Check sheet for the modelled part. Datum: model origin and axes. Units: mm. Face numbers are marked on the shaded views. A direction names the side the tool comes from. Round coordinates to 2 decimals unless told otherwise and drop trailing zeros. Write each loop counter-clockwise with the first axis right and the second up, starting at its lowest first coordinate (ties: lowest second). Pieces come first, ordered by that corner, then holes. Notation, with made-up numbers: (12.25, 75) - (31.25, 75) arc R21 ccw to (31.25, 81) - close; hole circle Ø3 at (-36.75, 62). An arc over 180 degrees is marked (long way). Answer as a JSON object with one key per item and string values. Group by question number.
Item 1: Gauge pin test, flat ends, axial feed: P1, Ø1.6, axis at x = -27.5, z = -8, coming from the +Y side; P2, Ø6, axis at x = -60, z = -7.5, coming from the +Y side. Record the tip position at first contact, or that the pin passes through.
Item 2: Release check for a two-part mould opening along X. For the marked faces 1, 2, 3 and 4 record: pulls with the +X half, pulls with the -X half, needs draft (parallel to the pull), parting line crosses it, or undercut.
Item 3: Sectioned sample at C-C on y = 3.75. Count the separate pieces of the cut face and the enclosed holes in it, plus the area to 3 significant figures.
Item 4: Sectioned sample at B-B on x = -7. Record the boundary of the cut face in (y, z), plus the area to 3 significant figures.
Item 5: Thickness scan on line 1 (X direction, y = 5.75, z = -28.5); line 2 (Z direction, x = -66, y = 9.25); line 3 (X direction, y = 7.25, z = -4.5). Record the ranges inside material, lowest first.
Item 6: Sectioned sample at D-D on x = -97. Record the boundary of the cut face in (y, z).
Item 7: Set-up check for the marked faces 5 and 6: record each of +Z, -Z, +X, -X, +Y, -Y from which the full face is reachable in a straight line by a thin tool's end or side.
Item 8: Sectioned sample at A-A on z = -46.4. Record the boundary of the cut face in (x, y).
```python
from build123d import *

# Parameters (mm, degrees)
SKETCH_1_W           = 120
SKETCH_1_H           = 53
EXTRUDE_2_DEPTH      = 16.4
SKETCH_4_W           = 116
SKETCH_4_H           = 49
CUT_EXTRUDE_5_DEPTH  = 15.2
SKETCH_5_W           = 118.4
SKETCH_5_H           = 51.4
CUT_EXTRUDE_6_DEPTH  = 3
SKETCH_6_W           = 57.1
SKETCH_6_H           = 36.3
EXTRUDE_3_DEPTH      = 10.7
SKETCH_7_W           = 55.5
SKETCH_7_H           = 35.5
CUT_EXTRUDE_7_DEPTH  = 10.7
SKETCH_8_W           = 3.401063497
SKETCH_8_H           = 16.4
CUT_EXTRUDE_8_DEPTH  = 10.7
SKETCH_9_R           = 8.9
EXTRUDE_4_DEPTH      = 14
SKETCH_10_R          = 7.7
CUT_EXTRUDE_9_DEPTH  = 14
SKETCH_12_W          = 1.431066628
SKETCH_12_H          = 20
CUT_EXTRUDE_10_DEPTH = 10.7
SKETCH_11_R          = 8
EXTRUDE_8_DEPTH      = 14
SKETCH_13_R          = 6.8
CUT_EXTRUDE_11_DEPTH = 14
SKETCH_14_W          = 22.6
SKETCH_14_H          = 8.7
EXTRUDE_9_DEPTH      = 12.2
SKETCH_15_W          = 21
SKETCH_15_H          = 9.750364289
CUT_EXTRUDE_12_DEPTH = 5.2
SKETCH_16_W          = 16
SKETCH_16_H          = 2
CUT_EXTRUDE_13_DEPTH = 7
SKETCH_18_W          = 21
SKETCH_18_H          = 2
CUT_EXTRUDE_14_DEPTH = 7
SKETCH_19_W          = 20.6
SKETCH_19_H          = 8.7
EXTRUDE_10_DEPTH     = 12.2
SKETCH_21_W          = 19
SKETCH_21_H          = 9.521560297
CUT_EXTRUDE_15_DEPTH = 5.2
SKETCH_23_W          = 16
SKETCH_23_H          = 2
CUT_EXTRUDE_16_DEPTH = 7
SKETCH_24_W          = 19
SKETCH_24_H          = 2
CUT_EXTRUDE_17_DEPTH = 7
SKETCH_25_R          = 1.2
CUT_EXTRUDE_18_DEPTH = 5
SKETCH_26_R          = 1.2
CUT_EXTRUDE_19_DEPTH = 5
SKETCH_27_R          = 1.2
CUT_EXTRUDE_20_DEPTH = 5
SKETCH_28_R          = 1.2
CUT_EXTRUDE_21_DEPTH = 5


with BuildPart() as part:
    # 草图1 → 凸台-拉伸2 (new body)
    with BuildSketch(Plane(origin=(0, 0, 0), x_dir=(1, 0, 0), z_dir=(0, 1, 0))):
        with Locations((-60, 26.5)):
            Rectangle(SKETCH_1_W, SKETCH_1_H)
    extrude(amount=EXTRUDE_2_DEPTH)

    # 草图4 → 切除-拉伸5 (cut)
    with BuildSketch(Plane(origin=(0, 16.4, 0), x_dir=(1, 0, 0), z_dir=(0, 1, 0))):
        with Locations((-60, 26.5)):
            Rectangle(SKETCH_4_W, SKETCH_4_H)
    extrude(amount=-CUT_EXTRUDE_5_DEPTH, mode=Mode.SUBTRACT)

    # 草图5 → 切除-拉伸6 (cut)
    with BuildSketch(Plane(origin=(0, 16.4, 0), x_dir=(1, 0, 0), z_dir=(0, 1, 0))):
        with Locations((-60, 26.5)):
            Rectangle(SKETCH_5_W, SKETCH_5_H)
    extrude(amount=-CUT_EXTRUDE_6_DEPTH, mode=Mode.SUBTRACT)

    # 草图6 → 凸台-拉伸3 (add)
    with BuildSketch(Plane(origin=(0, 1.2, 0), x_dir=(1, 0, 0), z_dir=(0, 1, 0))):
        with Locations((-58.55, 32.85)):
            Rectangle(SKETCH_6_W, SKETCH_6_H)
    extrude(amount=EXTRUDE_3_DEPTH)

    # 草图7 → 切除-拉伸7 (cut)
    with BuildSketch(Plane(origin=(0, 11.9, 0), x_dir=(1, 0, 0), z_dir=(0, 1, 0))):
        with Locations((-58.55, 33.25)):
            Rectangle(SKETCH_7_W, SKETCH_7_H)
    extrude(amount=-CUT_EXTRUDE_7_DEPTH, mode=Mode.SUBTRACT)

    # 草图8 → 切除-拉伸8 (cut)
    with BuildSketch(Plane(origin=(0, 11.9, 0), x_dir=(1, 0, 0), z_dir=(0, 1, 0))):
        with Locations((-86.528295274, 25.8)):
            Rectangle(SKETCH_8_W, SKETCH_8_H)
    extrude(amount=-CUT_EXTRUDE_8_DEPTH, mode=Mode.SUBTRACT)

    # 草图9 → 凸台-拉伸4 (add)
    with BuildSketch(Plane(origin=(0, 1.2, 0), x_dir=(1, 0, 0), z_dir=(0, 1, 0))):
        with Locations(Location((-97, 28, 0), (0, 0, 270))):
            Circle(SKETCH_9_R)
    extrude(amount=EXTRUDE_4_DEPTH)

    # 草图10 → 切除-拉伸9 (cut)
    with BuildSketch(Plane(origin=(0, 15.2, 0), x_dir=(1, 0, 0), z_dir=(0, 1, 0))):
        with Locations(Location((-97, 28, 0), (0, 0, 270))):
            Circle(SKETCH_10_R)
    extrude(amount=-CUT_EXTRUDE_9_DEPTH, mode=Mode.SUBTRACT)

    # 草图12 → 切除-拉伸10 (cut)
    with BuildSketch(Plane(origin=(0, 11.9, 0), x_dir=(1, 0, 0), z_dir=(0, 1, 0))):
        with Locations((-30.715533314, 27)):
            Rectangle(SKETCH_12_W, SKETCH_12_H)
    extrude(amount=-CUT_EXTRUDE_10_DEPTH, mode=Mode.SUBTRACT)

    # 草图11 → 凸台-拉伸8 (add)
    with BuildSketch(Plane(origin=(0, 1.2, 0), x_dir=(1, 0, 0), z_dir=(0, 1, 0))):
        with Locations(Location((-23, 28, 0), (0, 0, 270))):
            Circle(SKETCH_11_R)
    extrude(amount=EXTRUDE_8_DEPTH)

    # 草图13 → 切除-拉伸11 (cut)
    with BuildSketch(Plane(origin=(0, 15.2, 0), x_dir=(1, 0, 0), z_dir=(0, 1, 0))):
        with Locations(Location((-23, 28, 0), (0, 0, 270))):
            Circle(SKETCH_13_R)
    extrude(amount=-CUT_EXTRUDE_11_DEPTH, mode=Mode.SUBTRACT)

    # 草图14 → 凸台-拉伸9 (add)
    with BuildSketch(Plane(origin=(0, 1.2, 0), x_dir=(1, 0, 0), z_dir=(0, 1, 0))):
        with Locations((-23, 6.35)):
            Rectangle(SKETCH_14_W, SKETCH_14_H)
    extrude(amount=EXTRUDE_9_DEPTH)

    # 草图15 → 切除-拉伸12 (cut)
    with BuildSketch(Plane(origin=(0, 13.4, 0), x_dir=(1, 0, 0), z_dir=(0, 1, 0))):
        with Locations((-23, 6.875182145)):
            Rectangle(SKETCH_15_W, SKETCH_15_H)
    extrude(amount=-CUT_EXTRUDE_12_DEPTH, mode=Mode.SUBTRACT)

    # 草图16 → 切除-拉伸13 (cut)
    with BuildSketch(Plane(origin=(0, 16.4, 0), x_dir=(1, 0, 0), z_dir=(0, 1, 0))):
        with Locations((-23, 1)):
            Rectangle(SKETCH_16_W, SKETCH_16_H)
    extrude(amount=-CUT_EXTRUDE_13_DEPTH, mode=Mode.SUBTRACT)

    # 草图18 → 切除-拉伸14 (cut)
    with BuildSketch(Plane(origin=(0, 8.2, 0), x_dir=(1, 0, 0), z_dir=(0, 1, 0))):
        with Locations((-23, 8.5)):
            Rectangle(SKETCH_18_W, SKETCH_18_H)
    extrude(amount=-CUT_EXTRUDE_14_DEPTH, mode=Mode.SUBTRACT)

    # 草图19 → 凸台-拉伸10 (add)
    with BuildSketch(Plane(origin=(0, 1.2, 0), x_dir=(1, 0, 0), z_dir=(0, 1, 0))):
        with Locations((-97, 6.35)):
            Rectangle(SKETCH_19_W, SKETCH_19_H)
    extrude(amount=EXTRUDE_10_DEPTH)

    # 草图21 → 切除-拉伸15 (cut)
    with BuildSketch(Plane(origin=(0, 13.4, 0), x_dir=(1, 0, 0), z_dir=(0, 1, 0))):
        with Locations((-97, 6.760780149)):
            Rectangle(SKETCH_21_W, SKETCH_21_H)
    extrude(amount=-CUT_EXTRUDE_15_DEPTH, mode=Mode.SUBTRACT)

    # 草图23 → 切除-拉伸16 (cut)
    with BuildSketch(Plane(origin=(0, 16.4, 0), x_dir=(1, 0, 0), z_dir=(0, 1, 0))):
        with Locations((-97, 1)):
            Rectangle(SKETCH_23_W, SKETCH_23_H)
    extrude(amount=-CUT_EXTRUDE_16_DEPTH, mode=Mode.SUBTRACT)

    # 草图24 → 切除-拉伸17 (cut)
    with BuildSketch(Plane(origin=(0, 8.2, 0), x_dir=(1, 0, 0), z_dir=(0, 1, 0))):
        with Locations((-97, 8.5)):
            Rectangle(SKETCH_24_W, SKETCH_24_H)
    extrude(amount=-CUT_EXTRUDE_17_DEPTH, mode=Mode.SUBTRACT)

    # 草图25 → 切除-拉伸18 (cut)
    with BuildSketch(Plane(origin=(0, 1.2, 0), x_dir=(1, 0, 0), z_dir=(0, 1, 0))):
        with Locations(Location((-7, 7, 0), (0, 0, 270))):
            Circle(SKETCH_25_R)
    extrude(amount=-CUT_EXTRUDE_18_DEPTH, mode=Mode.SUBTRACT)

    # 草图26 → 切除-拉伸19 (cut)
    with BuildSketch(Plane(origin=(0, 1.2, 0), x_dir=(1, 0, 0), z_dir=(0, 1, 0))):
        with Locations(Location((-7, 46.4, 0), (0, 0, 270))):
            Circle(SKETCH_26_R)
    extrude(amount=-CUT_EXTRUDE_19_DEPTH, mode=Mode.SUBTRACT)

    # 草图27 → 切除-拉伸20 (cut)
    with BuildSketch(Plane(origin=(0, 1.2, 0), x_dir=(1, 0, 0), z_dir=(0, 1, 0))):
        with Locations(Location((-112.7, 7, 0), (0, 0, 270))):
            Circle(SKETCH_27_R)
    extrude(amount=-CUT_EXTRUDE_20_DEPTH, mode=Mode.SUBTRACT)

    # 草图28 → 切除-拉伸21 (cut)
    with BuildSketch(Plane(origin=(0, 1.2, 0), x_dir=(1, 0, 0), z_dir=(0, 1, 0))):
        with Locations(Location((-112.7, 46.4, 0), (0, 0, 270))):
            Circle(SKETCH_28_R)
    extrude(amount=-CUT_EXTRUDE_21_DEPTH, mode=Mode.SUBTRACT)


solid = part.part
```
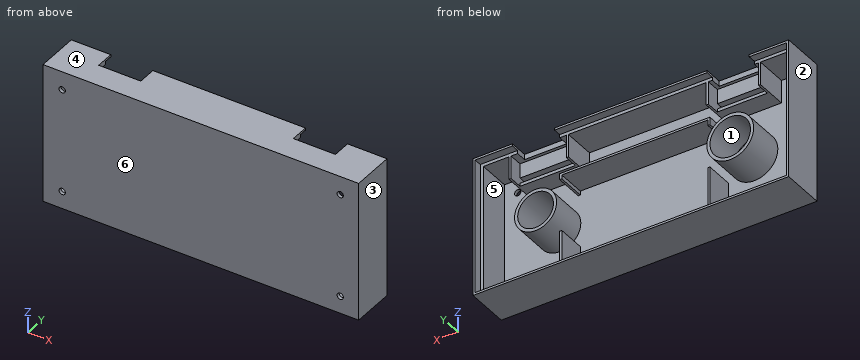
Completed:
{
 "1": {"P1": "y = 8.2", "P2": "y = 1.2"},
 "2": {"face 1": "undercut", "face 2": "pulls with the -X half", "face 3": "pulls with the +X half", "face 4": "needs draft"},
 "3": {"separate pieces": "4", "enclosed holes": "5", "area": "1,160 mm²"},
 "4": {"outline": "(0, -53) - (16.4, -53) - (16.4, -52.2) - (13.4, -52.2) - (13.4, -51) - (1.2, -51) - (1.2, -47.6) - (0, -47.6) - close; (0, -45.2) - (1.2, -45.2) - (1.2, -8.2) - (0, -8.2) - close; (0, -5.8) - (1.2, -5.8) - (1.2, -2) - (13.4, -2) - (13.4, -0.8) - (16.4, -0.8) - (16.4, 0) - (0, 0) - close", "area": "111 mm²"},
 "5": {"line 1": "-120 to -118, -105.89 to -104.68, -89.32 to -88.11, -30.98 to -29.78, -16.22 to -15.02, -2 to 0", "line 2": "-53 to -51, -15.5 to -14.7, -2 to 0", "line 3": "-120 to -118, -107.3 to -86.7, -34.3 to -11.7, -2 to 0"},
 "6": {"outline": "(0, -53) - (16.4, -53) - (16.4, -52.2) - (13.4, -52.2) - (13.4, -51) - (1.2, -51) - (1.2, -36.9) - (15.2, -36.9) - (15.2, -35.7) - (1.2, -35.7) - (1.2, -20.3) - (15.2, -20.3) - (15.2, -19.1) - (1.2, -19.1) - (1.2, -10.7) - (8.2, -10.7) - (8.2, -9.5) - (1.2, -9.5) - (1.2, -7.5) - (8.2, -7.5) - (8.2, -2) - (9.4, -2) - (9.4, 0) - (0, 0) - close"},
 "7": {"face 5": "+Y", "face 6": "+Z, -Z, +X, -X, -Y"},
 "8": {"outline": "(-120, 0) - (-113.9, 0) - (-113.9, 1.2) - (-118, 1.2) - (-118, 13.4) - (-119.2, 13.4) - (-119.2, 16.4) - (-120, 16.4) - close; (-111.5, 0) - (-8.2, 0) - (-8.2, 1.2) - (-30, 1.2) - (-30, 11.9) - (-30.8, 11.9) - (-30.8, 1.2) - (-86.3, 1.2) - (-86.3, 11.9) - (-87.1, 11.9) - (-87.1, 1.2) - (-111.5, 1.2) - close; (-5.8, 0) - (0, 0) - (0, 16.4) - (-0.8, 16.4) - (-0.8, 13.4) - (-2, 13.4) - (-2, 1.2) - (-5.8, 1.2) - close"}
}
